Read the model definition and answer for the solid it produces. Units are mm, in the model's axes. A direction names the side the tool comes from. Round coordinates to 2 decimals unless told otherwise and drop trailing zeros. Write each loop counter-clockwise with the first axis right and the second up, starting at its lowest first coordinate (ties: lowest second). Pieces come first, ordered by that corner, then holes. Notation, with made-up numbers: (85, 49) - (106, 49) arc R31 cw to (106, 77) - close; hole circle Ø6 at (88, 34). An arc over 180 degrees is marked (long way). Answer as CSV lines item,"result". Start each with the question number.
1) Consider line 1 along X through (y, z) = (29, 35); line 2 along Z through (x, y) = (19.5, 41.5); line 3 along Y through (x, z) = (22.5, 45). Determine where each line is inside the solid, lowest interval first.
2) Which of the six approach directions +Z, -Z, +X, -X, +Y, -Y give full straight-line access (tool end or side, diameter ignored) to faces 1 (the cylindrical face through (35.592, 22.108, 42.17)), 2 (the flat face through (25, 0, 25))?
3) This flat-tipped pin is pushed along its axis until it touches: pin 1 (10.5 mm diameter, centred on x = 22, y = 58, fed in from +Z). Where does it stop, or does it pass through?
4) Find section A-A on y = 50. Determine the outline of the cut face in (x, z), then the cut area to 3 significant figures.
5) Find section B-B on x = 20. Determine the outline of the cut face in (y, z).
6) For a pull along Y with two mould halves and no side action, classify faces 3 (the flat face through (24.895, 79.334, 42.39)), 4 (the flat face through (25, 100, 25)), 5 (the cylindrical face through (25.094, 77.085, 31.349)), 6 (the flat face through (25, 51, 0)) as +Y half, -Y half, draft (parallel to the pull), parting line (faces both ways), or undercut.
from build123d import *

# Parameters (mm, degrees)
SKIZZE1_W                       = 50
SKIZZE1_H                       = 100
AUFSATZ_LINEAR_AUSTRAGEN1_DEPTH = 50
SKIZZE2_W                       = 25
SKIZZE2_H                       = 60
SCHNITT_LINEAR_AUSTRAGEN1_DEPTH = 20
FORMSCHR_GE1_ANGLE              = 3
FORMSCHR_GE2_ANGLE              = 5
VERRUNDUNG1_R                   = 5


with BuildPart() as part:
    # Skizze1 → Aufsatz-Linear austragen1 (new body)
    with BuildSketch(Plane.XY):
        with Locations((25, 50)):
            Rectangle(SKIZZE1_W, SKIZZE1_H)
    extrude(amount=AUFSATZ_LINEAR_AUSTRAGEN1_DEPTH)

    # Skizze2 → Schnitt-Linear austragen1 (cut)
    with BuildSketch(Plane.XY.offset(50)):
        with Locations((25, 50)):
            Rectangle(SKIZZE2_W, SKIZZE2_H)
    extrude(amount=-SCHNITT_LINEAR_AUSTRAGEN1_DEPTH, mode=Mode.SUBTRACT)

    # Formschräge1
    formschr_ge1_faces = [part.faces().sort_by_distance(p)[0] for p in [
        (37.5, 50, 40),
        (12.5, 50, 40),
    ]]
    draft(formschr_ge1_faces, Plane.XY.offset(50), FORMSCHR_GE1_ANGLE)

    # Formschräge2
    formschr_ge2_faces = [part.faces().sort_by_distance(p)[0] for p in [
        (25, 20, 40.14586985),
        (25, 80, 40.14586985),
    ]]
    draft(formschr_ge2_faces, Plane.XY.offset(50), FORMSCHR_GE2_ANGLE)

    # Verrundung1
    verrundung1_edges = [part.edges().sort_by_distance(p)[0] for p in [
        (13.548155586, 50, 30),
        (13.024077793, 20.874886635, 40),
        (25, 78.250226729, 30),
        (13.024077793, 79.125113365, 40),
        (36.451844414, 50, 30),
        (36.975922207, 79.125113365, 40),
        (25, 21.749773271, 30),
        (36.975922207, 20.874886635, 40),
    ]]
    fillet(verrundung1_edges, radius=VERRUNDUNG1_R)


solid = part.part
Check values:
1,line 1,"x = 0 to 13.29, 36.71 to 50"
1,line 2,"z = 0 to 30"
1,line 3,"y = 0 to 20.44, 79.56 to 100"
2,face 1,"+Z"
2,face 2,"+Z, -Z, +X, -X, -Y"
3,pin 1,"stops at z = 30.24"
4,outline,"(0, 0) - (50, 0) - (50, 50) - (37.5, 50) - (36.7, 34.74) arc R5 cw to (31.71, 30) - (18.29, 30) arc R5 cw to (13.3, 34.74) - (12.5, 50) - (0, 50) - close"
4,area,"2,030 mm^2"
5,outline,"(0, 0) - (100, 0) - (100, 50) - (80, 50) - (78.65, 34.56) arc R5 cw to (73.67, 30) - (26.33, 30) arc R5 cw to (21.35, 34.56) - (20, 50) - (0, 50) - close"
6,face 3,"undercut"
6,face 4,"+Y half"
6,face 5,"undercut"
6,face 6,"draft"
